Model file for the job. Use its own axes, mm. A direction names the side the tool comes from. Give positions to 0.01 mm unless a question says otherwise; leave off trailing zeros. Write each loop counter-clockwise with the first axis right and the second up, starting at its lowest first coordinate (ties: lowest second). Pieces come first, ordered by that corner, then holes. Notation, with made-up numbers: (31.5, -3) - (40.5, -3) arc R18 cw to (40.5, 6) - close; hole circle Ø7 at (32.25, -31.5). An arc over 180 degrees is marked (long way). Use a Markdown table: item, result. Add a question column.
```python
from build123d import *

# Parameters (mm, degrees)
SKETCH_W     = 42
SKETCH_H     = 42
PAD_DEPTH    = 60
SKETCH001_R  = 21
PAD001_DEPTH = 35
SKETCH002_R  = 11
PAD002_DEPTH = 2
PAD003_DEPTH = 18
SKETCH004_R  = 2
POCKET_DEPTH = 6


with BuildPart() as part:
    # Sketch → Pad (new body)
    with BuildSketch(Plane.XY):
        with Locations((21, 21)):
            Rectangle(SKETCH_W, SKETCH_H)
    extrude(amount=PAD_DEPTH)

    # Sketch001 (on Face6 of Pad) → Pad001 (join)
    with BuildSketch(Plane.XY.offset(60)):
        with Locations((21, 21)):
            Circle(SKETCH001_R)
    extrude(amount=PAD001_DEPTH)

    # Sketch002 (on Face11 of Pad001) → Pad002 (join)
    with BuildSketch(Plane.XY.offset(95)):
        with Locations((21, 21)):
            Circle(SKETCH002_R)
    extrude(amount=PAD002_DEPTH)

    # Sketch003 (on Face13 of Pad002) → Pad003 (join)
    with BuildSketch(Plane.XY.offset(97)):
        with BuildLine():
            ThreePointArc((24, 23.645751), (17, 21), (24, 18.354249))
            Line((24, 23.645751), (24, 18.354249))
        make_face()
    extrude(amount=PAD003_DEPTH)

    # Sketch004 (on Face11 of Pad003) → Pocket (cut)
    with BuildSketch(Plane.XY.offset(95)):
        with Locations((10.393398, 10.393398)):
            Circle(SKETCH004_R)
        with Locations((31.606602, 10.393398)):
            Circle(SKETCH004_R)
        with Locations((31.606602, 31.606602)):
            Circle(SKETCH004_R)
        with Locations((10.393398, 31.606602)):
            Circle(SKETCH004_R)
    extrude(amount=-POCKET_DEPTH, mode=Mode.SUBTRACT)


solid = part.part
```
(1) Two-plate mould, pull along X, no slides. Class faces 5 (the flat face through (24, 21, 106)), 6 (the flat face through (32, 10, 89)), 7 (the flat face through (26, 21, 97)), 8 (the cylindrical face through (30.133, 32.958, 92.042)): +X half, -X half, draft (parallel to the pull), parting line (faces both ways), or undercut.
(2) Band-saw the part on C-C (z = 71). Write the cut outline in (x, y).
(3) Band-saw the part on B-B (x = 4.5). Write the cut outline in (y, z).
(4) Band-saw the part on A-A (y = 36.5). Write the cut outline in (x, z), then the cut area to 3 significant figures.
(5) Probe probe 1 along Y at (x, z) = (21, 110.5); probe 2 along Z at (x, y) = (32.5, 19.5); probe 3 along Z at (x, y) = (15.5, 13). List the from-to ranges inside material, lowest first. Write a range as [from, to].
(6) Which spindle directions (+Z, -Z, +X, -X, +Y, -Y) get a long thin tool onto all of the face, cutting with end or side? Do faces 1 (the flat face through (4, 37, 60)), 2 (the flat face through (37, 38, 60)), 3 (the flat face through (38, 4, 60)), 4 (the flat face through (32, 32, 89)). Say none if no direction does.
(7) Flat gauge pins, fed straight in: pin 1 (10 mm diameter, centred on y = 9, z = 84, fed in from +X); pin 2 (3 mm diameter, centred on x = 31.5, y = 32.5, fed in from +Z); pin 3 (5 mm diameter, centred on x = 27.5, z = 57.5, fed in from -Y); pin 4 (10.5 mm diameter, centred on x = 15, y = 7.5, fed in from +Z). Where does each tip first touch, or does it go through?
Model answer:
| question | item | result |
|---|---|---|
| 1 | face 5 | +X half |
| 1 | face 6 | undercut |
| 1 | face 7 | draft |
| 1 | face 8 | undercut |
| 2 | outline | circle Ø42 at (21, 21) |
| 3 | outline | (0, 0) - (42, 0) - (42, 60) - (33.99, 60) - (33.99, 95) - (8.01, 95) - (8.01, 60) - (0, 60) - close |
| 4 | outline | (0, 0) - (42, 0) - (42, 60) - (35.17, 60) - (35.17, 95) - (6.83, 95) - (6.83, 60) - (0, 60) - close |
| 4 | area | 3,510 mm^2 |
| 5 | probe 1 | y = [17, 25] |
| 5 | probe 2 | z = [0, 95] |
| 5 | probe 3 | z = [0, 97] |
| 6 | face 1 | +Z, -X, +Y |
| 6 | face 2 | +Z, +X, +Y |
| 6 | face 3 | +Z, +X, -Y |
| 6 | face 4 | +Z |
| 7 | pin 1 | stops at x = 40.8 |
| 7 | pin 2 | stops at z = 95 |
| 7 | pin 3 | stops at y = 0 |
| 7 | pin 4 | stops at z = 97 |
